```python
from build123d import *

# Parameters (mm, degrees)
F0_W          = 95.25
F0_H          = 101.6
F1_DEPTH      = 95.25
F2_W          = 69.85
F2_H          = 304.8
F3_DEPTH      = 95.251
F3_DEPTH_BACK = 95.251
F5_SIZE       = 25.4
F6_SIZE       = 25.4
F8_DEPTH      = 25.4


with BuildPart() as f1:
    # F0 (on Front) → F1 (new body, symmetric)
    with BuildSketch(Plane.XZ):
        with Locations((47.625, -50.8)):
            Rectangle(F0_W, F0_H)
        with Locations((-47.625, -50.8)):
            Rectangle(F0_W, F0_H)
        Polygon((95.25, 203.2), (-95.25, 203.2), (-95.25, 0), (0, 0), (95.25, 0), align=None)
        Polygon((33.3162687146, 858.8361700868), (0, 872.7179487179), (-33.3162687146, 858.8361700868), (-69.85, 843.6137820513), (-95.25, 833.0304487179), (-95.25, 203.2), (95.25, 203.2), (95.25, 833.0304487179), (69.85, 843.6137820513), align=None)
        Polygon((0, 872.7179487179), (0, 1092.8512820513), (-58.7162687146, 1068.3861700868), (-33.3162687146, 858.8361700868), align=None)
        Polygon((58.7162687146, 1068.3861700868), (0, 1092.8512820513), (0, 872.7179487179), (33.3162687146, 858.8361700868), align=None)
        Polygon((-33.3162687146, 858.8361700868), (-58.7162687146, 1068.3861700868), (-69.85, 1063.7471153846), (-69.85, 843.6137820513), align=None)
        Polygon((69.85, 1063.7471153846), (58.7162687146, 1068.3861700868), (33.3162687146, 858.8361700868), (69.85, 843.6137820513), align=None)
        Polygon((-69.85, 1063.7471153846), (-95.25, 1053.1637820513), (-69.85, 843.6137820513), align=None)
        Polygon((69.85, 843.6137820513), (95.25, 1053.1637820513), (69.85, 1063.7471153846), align=None)
    extrude(amount=F1_DEPTH, both=True)

    # F2 (on Right) → F3 (cut, two sides)
    with BuildSketch(Plane.YZ) as f3_sk:
        with Locations((-60.325, 50.8)):
            Rectangle(F2_W, F2_H)
        with Locations((60.325, 50.8)):
            Rectangle(F2_W, F2_H)
    extrude(amount=-F3_DEPTH, mode=Mode.SUBTRACT)
    extrude(f3_sk.sketch, amount=F3_DEPTH_BACK, mode=Mode.SUBTRACT)

    # F5
    f5_edges = [f1.edges().sort_by_distance(p)[0] for p in [
        (95.25, 0, -101.6),
    ]]
    chamfer(f5_edges, length=F5_SIZE)

    # F6
    f6_edges = [f1.edges().sort_by_distance(p)[0] for p in [
        (-95.25, 0, -101.6),
    ]]
    chamfer(f6_edges, length=F6_SIZE)

    # F7 (on Front) → F8 (cut, symmetric)
    with BuildSketch(Plane.XZ):
        Polygon((58.7162687146, 1068.3861700868), (33.3162687146, 858.8361700868), (69.85, 843.6137820513), (95.25, 1053.1637820513), align=None)
        Polygon((-33.3162687146, 858.8361700868), (-58.7162687146, 1068.3861700868), (-95.25, 1053.1637820513), (-69.85, 843.6137820513), align=None)
    extrude(amount=F8_DEPTH, both=True, mode=Mode.SUBTRACT)


solid = f1.part
```
Model file for the job. Use its own axes, mm. A direction names the side the tool comes from. Give positions to 0.01 mm unless a question says otherwise; leave off trailing zeros. Write each loop counter-clockwise with the first axis right and the second up, starting at its lowest first coordinate (ties: lowest second). Pieces come first, ordered by that corner, then holes. Notation, with made-up numbers: (-4.5, 45) -> (17.5, 45) arc R21 ccw to (17.5, 49) -> close; hole circle Ø10 at (41, 37.25). An arc over 180 degrees is marked (long way). Use CSV: the item, a comma, the result in double quotes. Start each with the question number.
1) Pin check, flat tips, straight feed: P1, Ø21, axis at x = 34.5, y = -48.5, coming from the -Z side; P2, Ø6, axis at x = 16.5, y = -30, coming from the +Z side; P3, Ø2, axis at x = 73, z = 849.5, coming from the -Y side. Stop position of each tip, or through.
2) Cut at A-A on y = 76. List the corners of the cut face in (x, z), plus the area to 3 significant figures.
3) Tool access for faces 1 (the flat face through (64, 25.4, 958)), 2 (the flat face through (-65, -25.4, 958)), 3 (the flat face through (1, -25.4, 49)): list every direction of +Z, -Z, +X, -X, +Y, -Y with a clear straight run to the whole face (end or side of a thin tool).
4) Cut at C-C on z = 37.5. List the corners of the cut face in (x, y).
5) Drill centre lines: L1, parallel to Y at x = 79, z = 945; L2, parallel to Y at x = -65.5, z = 119; L3, parallel to Z at x = -70, y = 4.5. Where is each one in solid material? Low to high.
6) Cut at D-D on y = 6. List the corners of the cut face in (x, z), plus the area to 3 significant figures.
7) Two-plate mould, pull along Z, no slides. Class faces 4 (the flat face through (-1, 0, -101.6)), 5 (the flat face through (-65, 25.4, 958)), 6 (the flat face through (-95.25, -1, 486)): released by +Z, released by -Z, zero draft, split by the parting line, or undercut.
8) Cut at B-B on x = -23. List the corners of the cut face in (y, z).
Final values:
1,P1,"stops at z = 203.2"
1,P2,"stops at z = 1087.23"
1,P3,"passes through"
2,outline,"(-95.25, 203.2) -> (95.25, 203.2) -> (95.25, 833.03) -> (69.85, 843.61) -> (95.25, 1053.16) -> (0, 1092.85) -> (-95.25, 1053.16) -> (-69.85, 843.61) -> (-95.25, 833.03) -> close"
2,area,"160,000 mm2"
3,face 1,"+X"
3,face 2,"-X"
3,face 3,"-Z, +X, -X, -Y"
4,outline,"(-95.25, -25.4) -> (95.25, -25.4) -> (95.25, 25.4) -> (-95.25, 25.4) -> close"
5,L1,"y = -95.25 to -25.4, 25.4 to 95.25"
5,L2,"y = -25.4 to 25.4"
5,L3,"z = -101.45 to 843.55"
6,outline,"(-95.25, -76.2) -> (-69.85, -101.6) -> (69.85, -101.6) -> (95.25, -76.2) -> (95.25, 833.03) -> (33.32, 858.84) -> (58.72, 1068.39) -> (0, 1092.85) -> (-58.72, 1068.39) -> (-33.32, 858.84) -> (-95.25, 833.03) -> close"
6,area,"201,000 mm2"
7,face 4,"released by -Z"
7,face 5,"undercut"
7,face 6,"zero draft"
8,outline,"(-95.25, 203.2) -> (-25.4, 203.2) -> (-25.4, -101.6) -> (25.4, -101.6) -> (25.4, 203.2) -> (95.25, 203.2) -> (95.25, 1083.27) -> (-95.25, 1083.27) -> close"
